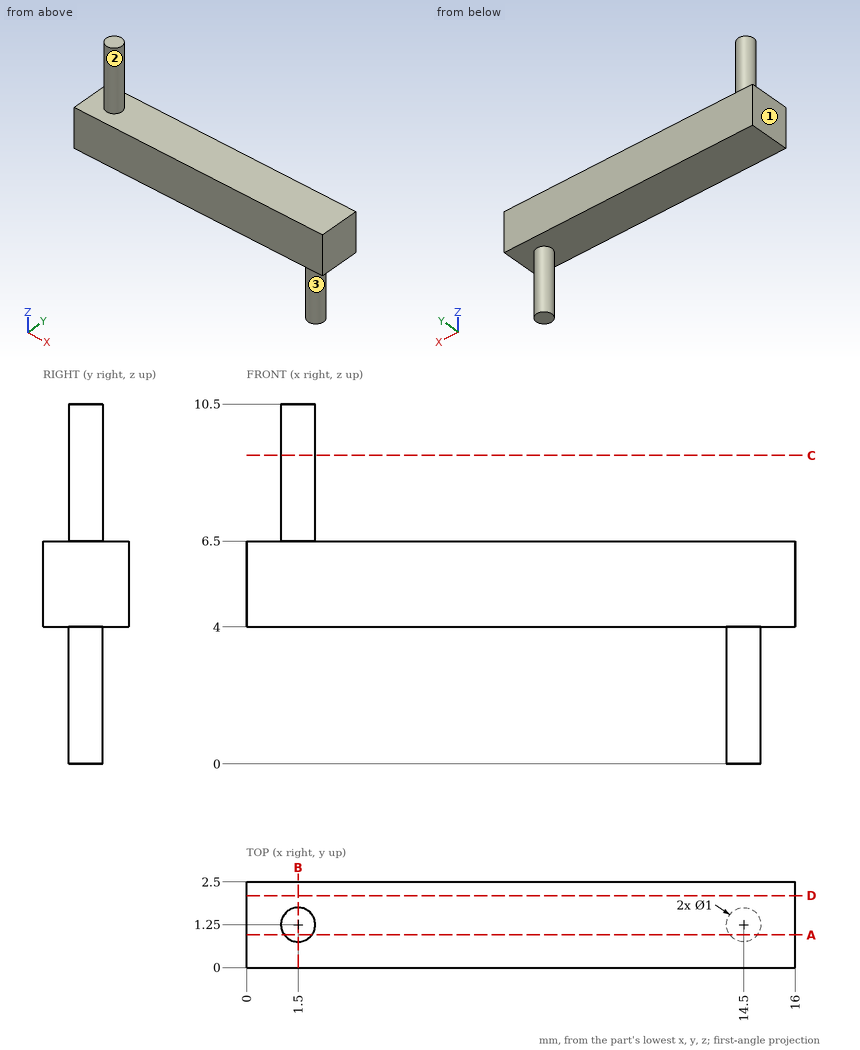
Part print with two shaded views. Sizes in mm from the minimum x, y, z corner. A direction names the side the tool comes from. Round coordinates to 2 decimals unless told otherwise and drop trailing zeros. Order: outer loops, then holes, each group sorted by start corner. A loop starts at its lowest first (then second) coordinate and runs counter-clockwise, first axis right, second up. Notation, with made-up numbers: M 40,59.5 L 57,59.5 A24 ccw 57,83.5 Z; hole C -13.5,37.25 d3. An arc over 180 degrees is marked long. Answer in a Markdown table with one row per item. Add a question column.
Q1. Wall check: L1, parallel to Z at x = 10.5, y = 2.25; L2, parallel to X at y = 1.1, z = 3.5; L3, parallel to X at y = 1.6, z = 8.5. Give the ranges that are in metal, low to high. Write a range as from..to.
Q2. Cut at D-D on y = 2.1. Give the cut face in (x, z).
Q3. Cut at C-C on z = 9. Give the cut face in (x, y).
Q4. Cut at A-A on y = 0.95. Give the cut face in (x, z), and give its area (3 significant figures).
Q5. Cut at B-B on x = 1.5. Give the cut face in (y, z).
Q6. Pin check, flat tips, straight feed: pin 1 (1 mm diameter, centred on x = 10.5, y = 1, fed in from +Z); pin 2 (1.2 mm diameter, centred on x = 4, y = 1.5, fed in from -Z). Stop position of each tip, or through.
Q7. 3-axis set-ups, long thin cutter, end or side, ignore diameter. For the marked faces 1, 2 and 3: which of +Z, -Z, +X, -X, +Y, -Y reach the whole face in a straight line?
Established:
| question | item | result |
|---|---|---|
| 1 | L1 | z = 4..6.5 |
| 1 | L2 | x = 14.02..14.98 |
| 1 | L3 | x = 1.14..1.86 |
| 2 | outline | M 0,4 L 16,4 L 16,6.5 L 0,6.5 Z |
| 3 | outline | C 1.5,1.25 d1 |
| 4 | outline | M 0,4 L 14.1,4 L 14.1,0 L 14.9,0 L 14.9,4 L 16,4 L 16,6.5 L 1.9,6.5 L 1.9,10.5 L 1.1,10.5 L 1.1,6.5 L 0,6.5 Z |
| 4 | area | 46.4 mm2 |
| 5 | outline | M 0,4 L 2.5,4 L 2.5,6.5 L 1.75,6.5 L 1.75,10.5 L 0.75,10.5 L 0.75,6.5 L 0,6.5 Z |
| 6 | pin 1 | stops at z = 6.5 |
| 6 | pin 2 | stops at z = 4 |
| 7 | face 1 | +Z, -Z, -X, +Y, -Y |
| 7 | face 2 | +Z |
| 7 | face 3 | -Z |
